from build123d import *

# Parameters (mm, degrees)
SKETCH1_W           = 50.8
SKETCH1_H           = 25.4
SKETCH1_W_2         = 44.45
SKETCH1_H_2         = 19.05
BOSS_EXTRUDE1_DEPTH = 457.2
SKETCH2_R           = 4.7625
CUT_EXTRUDE1_DEPTH  = 461.188841673
SKETCH3_W           = 50.8
SKETCH3_H           = 25.4
SKETCH3_W_2         = 44.45
SKETCH3_H_2         = 19.05
BOSS_EXTRUDE2_DEPTH = 76.2
SKETCH4_R           = 4.7625
CUT_EXTRUDE2_DEPTH  = 536.964075289


with BuildPart() as part:
    # Sketch1 → Boss-Extrude1 (new body)
    with BuildSketch(Plane.XY):
        Rectangle(SKETCH1_W, SKETCH1_H)
        Rectangle(SKETCH1_W_2, SKETCH1_H_2, mode=Mode.SUBTRACT)
    extrude(amount=BOSS_EXTRUDE1_DEPTH)

    # Sketch2 → Cut-Extrude1 (cut, through all)
    with BuildSketch(Plane.ZY.offset(25.4)):
        with Locations((438.15, 0)):
            Circle(SKETCH2_R)
    extrude(amount=-CUT_EXTRUDE1_DEPTH, mode=Mode.SUBTRACT)

    # Sketch3 → Boss-Extrude2 (add)
    with BuildSketch(Plane.XY.offset(457.2)):
        Rectangle(SKETCH3_W, SKETCH3_H)
        Rectangle(SKETCH3_W_2, SKETCH3_H_2, mode=Mode.SUBTRACT)
    extrude(amount=BOSS_EXTRUDE2_DEPTH)

    # Sketch4 → Cut-Extrude2 (cut, through all)
    with BuildSketch(Plane.ZY.offset(25.4)):
        with Locations((520.7, 0)):
            Circle(SKETCH4_R)
    extrude(amount=-CUT_EXTRUDE2_DEPTH, mode=Mode.SUBTRACT)


solid = part.part
Source: CAD feature listing. Evaluate the final solid. Frame: model axes, mm. A direction names the side the tool comes from. Coordinates: 2 decimals unless noted, no trailing zeros. Loops run counter-clockwise (first coordinate to the right, second up) from the corner with the lowest first, then second, coordinate; pieces in that order, holes last. Notation, with made-up numbers: (34, 44.25) - (81, 44.25) arc R36 cw to (81, 79.25) - close; hole circle Ø5 at (44.5, 4.5). An arc over 180 degrees is marked (long way). Return JSON: item names as keys, results as strings.
Q1. Section A-A, the plane z = 438.15. Return loops of the section in (x, y) (1 decimal).
Results:
{"outline": "(-25.4, -12.7) - (25.4, -12.7) - (25.4, -4.8) - (22.2, -4.8) - (22.2, -9.5) - (-22.2, -9.5) - (-22.2, -4.8) - (-25.4, -4.8) - close; (-25.4, 4.8) - (-22.2, 4.8) - (-22.2, 9.5) - (22.2, 9.5) - (22.2, 4.8) - (25.4, 4.8) - (25.4, 12.7) - (-25.4, 12.7) - close"}
Q2. Material intervals for line 1 along Y through (x, z) = (16, 219) (3 decimals); line 2 along Y through (x, z) = (-23.3, 520.7); line 3 along X through (y, z) = (4, 414) (3 decimals), sorted ascending.
Results:
{"line 1": "-12.7 to -9.525, 9.525 to 12.7", "line 2": "-12.7 to -4.76, 4.76 to 12.7", "line 3": "-25.4 to -22.225, 22.225 to 25.4"}
Q3. Section C-C, the plane y = 0. Return loops of the section in (x, z) (1 decimal), plus the area to 3 significant figures.
Results:
{"outline": "(-25.4, 0) - (-22.2, 0) - (-22.2, 433.4) - (-25.4, 433.4) - close; (-25.4, 442.9) - (-22.2, 442.9) - (-22.2, 515.9) - (-25.4, 515.9) - close; (-25.4, 525.5) - (-22.2, 525.5) - (-22.2, 533.4) - (-25.4, 533.4) - close; (22.2, 0) - (25.4, 0) - (25.4, 433.4) - (22.2, 433.4) - close; (22.2, 442.9) - (25.4, 442.9) - (25.4, 515.9) - (22.2, 515.9) - close; (22.2, 525.5) - (25.4, 525.5) - (25.4, 533.4) - (22.2, 533.4) - close", "area": "3,270 mm2"}
Q4. Section D-D, the plane z = 190.5. Return loops of the section in (x, y) (3 decimals).
Results:
{"outline": "(-25.4, -12.7) - (25.4, -12.7) - (25.4, 12.7) - (-25.4, 12.7) - close; hole (-22.225, -9.525) - (22.225, -9.525) - (22.225, 9.525) - (-22.225, 9.525) - close"}
Q5. Mould query, pull axis X, two halves, no side actions, for faces 3 (the flat face through (0, 10, 533.4)), 4 (the flat face through (25.4, 0, 263)), 5 (the flat face through (0, -9.525, 263)). Classes: released by +X, released by -X, zero draft, split by the parting line, or undercut.
Results:
{"face 3": "zero draft", "face 4": "released by +X", "face 5": "undercut"}
Q6. Section B-B, the plane x = 4. Return loops of the section in (y, z) (3 decimals), plus the area to 3 significant figures.
Results:
{"outline": "(-12.7, 0) - (-9.525, 0) - (-9.525, 533.4) - (-12.7, 533.4) - close; (9.525, 0) - (12.7, 0) - (12.7, 533.4) - (9.525, 533.4) - close", "area": "3,390 mm2"}
Q7. Access query for faces 1 (the flat face through (-25.4, 0, 263)), 2 (the flat face through (22.225, 0, 263)). Directions: +Z, -Z, +X, -X, +Y, -Y. A direction counts if a zero-diameter tool reaches every point of the face in a straight line with its end or side. Return the directions, or none.
Results:
{"face 1": "+Z, -Z, -X, +Y, -Y", "face 2": "+Z, -Z"}
